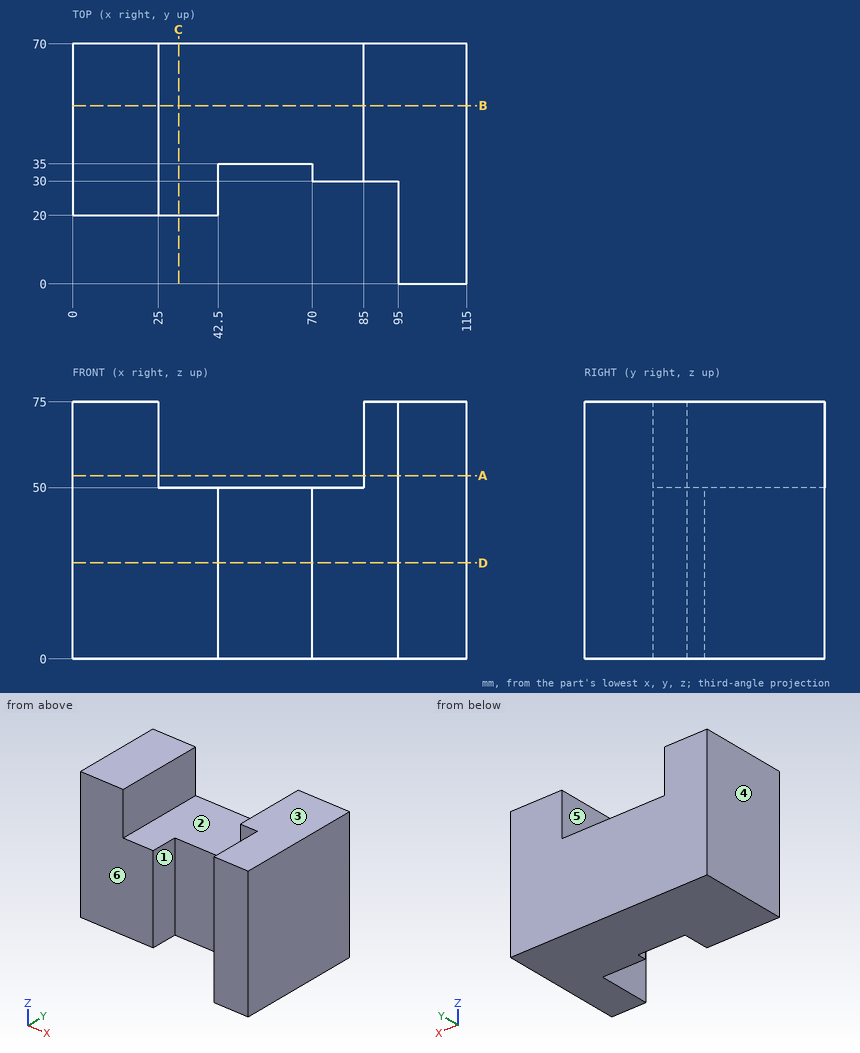
Design review of the part shown in the three views and the two pictorial views. Dimensions are in mm from the part's minimum x, y and z. A direction names the side the tool comes from. Give positions to 0.01 mm unless a question says otherwise; leave off trailing zeros. Loops run counter-clockwise (first coordinate to the right, second up) from the corner with the lowest first, then second, coordinate; pieces in that order, holes last. Notation, with made-up numbers: M -10,3.25 L 12,3.25 A20 cw 12,25.25 Z; hole C 5.25,71 d7. An arc over 180 degrees is marked long. Answer as a JSON object with one key per item and string values.
Item 1: We need section A-A (z = 53.5). State the section outline as (x, y) points, and give its area (3 significant figures).
Output values:
{"outline": "M 0,20 L 25,20 L 25,70 L 0,70 Z; M 85,30 L 95,30 L 95,0 L 115,0 L 115,70 L 85,70 Z", "area": "3,050 mm2"}
Item 2: Wall thickness on line 1 along X through (y, z) = (60.5, 54.5); line 2 along X through (y, z) = (25, 60.5); line 3 along Y through (x, z) = (59.5, 28): over which ranges is each line inside the solid? List them lowest first.
Output values:
{"line 1": "x = 0 to 25, 85 to 115", "line 2": "x = 0 to 25, 95 to 115", "line 3": "y = 35 to 70"}
Item 3: For P1, Ø12.5, axis at x = 86.5, z = 25.5, coming from the -Y side; P2, Ø3, axis at x = 32, y = 20.5, coming from the +Z side; P3, Ø14, axis at x = 54, z = 34.5, coming from the -Y side, all flat-tipped, find the tip position at first contact; note any pin that passes through.
Output values:
{"P1": "stops at y = 30", "P2": "stops at z = 50", "P3": "stops at y = 35"}
Item 4: Machinability: for the marked faces 1, 2 and 3, which of the approach directions +Z, -Z, +X, -X, +Y, -Y give a long, thin tool a straight path to every point of the face, cutting with its end or side? Answer none if there is none.
Output values:
{"face 1": "+Z, -Z, -Y", "face 2": "+Z, +Y, -Y", "face 3": "+Z, +X, -X, +Y, -Y"}
Item 5: We need section B-B (y = 52). State the section outline as (x, z) points.
Output values:
{"outline": "M 0,0 L 115,0 L 115,75 L 85,75 L 85,50 L 25,50 L 25,75 L 0,75 Z"}
Item 6: We need section C-C (x = 31). State the section outline as (y, z) points.
Output values:
{"outline": "M 20,0 L 70,0 L 70,50 L 20,50 Z"}
Item 7: We need section D-D (z = 28). State the section outline as (x, y) points.
Output values:
{"outline": "M 0,20 L 42.5,20 L 42.5,35 L 70,35 L 70,30 L 95,30 L 95,0 L 115,0 L 115,70 L 0,70 Z"}
Item 8: Mouldability with a two-part tool opening along X and no side actions: class the marked faces 4, 5 and 6 as pulls with the +X half, pulls with the -X half, needs draft (parallel to the pull), parting line crosses it, or undercut.
Output values:
{"face 4": "pulls with the -X half", "face 5": "undercut", "face 6": "needs draft"}
